Here's how the part is built. I have some questions about the finished solid (model axes, mm). A direction names the side the tool comes from. Round coordinates to 2 decimals unless told otherwise and drop trailing zeros. Write each loop counter-clockwise with the first axis right and the second up, starting at its lowest first coordinate (ties: lowest second). Pieces come first, ordered by that corner, then holes. Notation, with made-up numbers: (39.25, -37) -> (71.25, -37) arc R22 ccw to (71.25, -9) -> close; hole circle Ø2 at (68, 18). An arc over 180 degrees is marked (long way). Answer in a Markdown table with one row per item.
from build123d import *

# Parameters (mm, degrees)
ESBO_O1_W                                            = 18
ESBO_O1_H                                            = 28.5
RESSALTO_EXTRUS_O1_DEPTH                             = 8
ESCAREADO_PARA_PARAFUSO_COM_CABE_A_ESCAR_D           = 2.4
ESCAREADO_PARA_PARAFUSO_COM_CABE_A_ESCAR_CSINK_D     = 4.4
ESCAREADO_PARA_PARAFUSO_COM_CABE_A_ESCAR_CSINK_ANGLE = 90
CORTE_EXTRUS_O1_DEPTH                                = 4
ESCAREADO_PARA_PARAFUSO_COM_CABE_A_E_3_D             = 2.4
ESCAREADO_PARA_PARAFUSO_COM_CABE_A_E_3_CSINK_D       = 4.4
ESCAREADO_PARA_PARAFUSO_COM_CABE_A_E_3_CSINK_ANGLE   = 90
CORTE_EXTRUS_O2_DEPTH                                = 35.644624403
FILETE1_R                                            = 5
CHANFRO1_SIZE                                        = 1
CHANFRO2_SIZE                                        = 1
BROCA_DE_ROSQUEAR_PARA_TARRAXA_DE_M21_D              = 1.6


# Read off the part's stored shape, not the designer's step: Escareado para parafuso com cabeça escareada chata de M21
with BuildPart() as part:
    # Esboço1 → Ressalto-extrusão1 (new body)
    with BuildSketch(Plane(origin=(0, 0, 0), x_dir=(1, 0, 0), z_dir=(0, 1, 0))):
        with Locations((9, 14.25)):
            Rectangle(ESBO_O1_W, ESBO_O1_H)
        with BuildLine():
            Line((5, 11.5), (13, 11.5))
            ThreePointArc((13, 11.5), (14.414213562, 12.085786438), (15, 13.5))
            Line((15, 13.5), (15, 16.5))
            ThreePointArc((15, 16.5), (14.414213562, 17.914213562), (13, 18.5))
            Line((13, 18.5), (5, 18.5))
            ThreePointArc((5, 18.5), (3.585786438, 17.914213562), (3, 16.5))
            Line((3, 16.5), (3, 13.5))
            ThreePointArc((3, 13.5), (3.585786438, 12.085786438), (5, 11.5))
        make_face(mode=Mode.SUBTRACT)
    extrude(amount=RESSALTO_EXTRUS_O1_DEPTH)

    # Escareado para parafuso com cabe_a escar (through all)
    with Locations(Plane(origin=(5, 8, -26), x_dir=(0, 0, 1), z_dir=(0, 1, 0))):
        with Locations((0, 0), (0, 8)):
            CounterSinkHole(ESCAREADO_PARA_PARAFUSO_COM_CABE_A_ESCAR_D / 2, ESCAREADO_PARA_PARAFUSO_COM_CABE_A_ESCAR_CSINK_D / 2, counter_sink_angle=ESCAREADO_PARA_PARAFUSO_COM_CABE_A_ESCAR_CSINK_ANGLE)

    # Esboço10 → Corte-extrusão1 (cut)
    with BuildSketch(Plane.XZ):
        Polygon((0, -28.5), (18, -28.5), (18, -23.5), (15, -23.5), (15, -15), (3, -15), (3, -23.5), (0, -23.5), align=None)
    extrude(amount=-CORTE_EXTRUS_O1_DEPTH, mode=Mode.SUBTRACT)

    # Escareado para parafuso com cabe_a e 2 o → Escareado para parafuso com cabe_a e 2 (revolve, cut)
    with BuildSketch(Plane(origin=(0, 2, -21.5), x_dir=(0, 1, 0), z_dir=(0, 0, -1))):
        Polygon((2.2, 18), (0, 18), (0, 15), (1.2, 15), (1.2, 17), align=None)
    revolve(axis=Axis((0, 2, -21.5), (1, 0, 0)), mode=Mode.SUBTRACT)

    # Escareado para parafuso com cabe_a e 3 (through all)
    with Locations(Plane(origin=(0, 2, -21.5), x_dir=(0, 0, -1), z_dir=(-1, 0, 0))):
        with Locations((0, 0)):
            CounterSinkHole(ESCAREADO_PARA_PARAFUSO_COM_CABE_A_E_3_D / 2, ESCAREADO_PARA_PARAFUSO_COM_CABE_A_E_3_CSINK_D / 2, counter_sink_angle=ESCAREADO_PARA_PARAFUSO_COM_CABE_A_E_3_CSINK_ANGLE)

    # Esboço15 → Corte-extrusão2 (cut, through all)
    with BuildSketch(Plane(origin=(0, 8, 0), x_dir=(1, 0, 0), z_dir=(0, 1, 0))):
        Polygon((0, 0), (4, 0), (0, 11.5), align=None)
        Polygon((18, 0), (18, 11.5), (14, 0), align=None)
    extrude(amount=-CORTE_EXTRUS_O2_DEPTH, mode=Mode.SUBTRACT)

    # Filete1
    filete1_edges = [part.edges().sort_by_distance(p)[0] for p in [
        (0, 4, -11.5),
        (4, 4, 0),
        (14, 4, 0),
        (18, 4, -11.5),
    ]]
    fillet(filete1_edges, radius=FILETE1_R)

    # Chanfro1
    chanfro1_edges = [part.edges().sort_by_distance(p)[0] for p in [
        (16.445137101, 8, -7.029769164),
        (0, 8, -20.422372289),
        (1.554862899, 8, -7.029769164),
        (9, 8, 0),
        (18, 8, -20.422372289),
        (13.342458661, 8, -0.924891681),
        (0.069867146, 8, -11.511803979),
        (4.657541339, 8, -0.924891681),
        (17.930132854, 8, -11.511803979),
        (3.585786438, 8, -12.085786438),
        (14.414213562, 8, -17.914213562),
        (9, 8, -18.5),
        (3.585786438, 8, -17.914213562),
        (3, 8, -15),
        (9, 8, -11.5),
        (14.414213562, 8, -12.085786438),
        (15, 8, -15),
    ]]
    chamfer(chanfro1_edges, length=CHANFRO1_SIZE)

    # Chanfro2
    # the kernel refuses this chamfer: 1 mm, written as the material it takes off along each edge
    with BuildSketch(Plane(origin=(0, 0, -26.071682988), x_dir=(0.9996219169112968, -0.027495876610586372, 0), z_dir=(0, 0, 1)), Plane(origin=(18, 0, -19.844832151), x_dir=(-0.9996219169112968, -0.02749587661058639, 0), z_dir=(0, 0, -1))) as chanfro2_piece_1:
        Polygon((CHANFRO2_SIZE * 0.999621916911, CHANFRO2_SIZE * 0.0274958766106), (-CHANFRO2_SIZE * 0.0274958766106, CHANFRO2_SIZE * 0.999621916911), (0, 0), align=None)
    extrude(amount=6.226850837, mode=Mode.SUBTRACT)
    with BuildSketch(Plane(origin=(17.722483984, 0, -10.702141453), x_dir=(-0.94413969843999, -0.02749587661058639, -0.32839641684869236), z_dir=(-0.3285206249412729, 0, 0.944496796706159)), Plane(origin=(2.832209783, 0, -3.357396875), x_dir=(0.9441396984399901, -0.02749587661058552, -0.32839641684869225), z_dir=(-0.32852062494127277, 0, -0.9444967967061592))) as chanfro2_piece_2:
        Polygon((CHANFRO2_SIZE * 0.999621916911, -CHANFRO2_SIZE * 0.0274958766106), (-CHANFRO2_SIZE * 0.0274958766106, -CHANFRO2_SIZE * 0.999621916911), (0, 0), align=None)
    extrude(amount=7.776357318, mode=Mode.SUBTRACT)
    with BuildSketch(Plane(origin=(18, 0, -12.344744577), x_dir=(-0.9996219169112968, -0.02749587661058639, 0), z_dir=(0, 0, -1)), Plane(origin=(0, 0, -23.155167849), x_dir=(0.9996219169112968, -0.027495876610586372, 0), z_dir=(0, 0, 1))) as chanfro2_piece_3:
        Polygon((CHANFRO2_SIZE * 0.999621916911, CHANFRO2_SIZE * 0.0274958766106), (-CHANFRO2_SIZE * 0.0274958766106, CHANFRO2_SIZE * 0.999621916911), (0, 0), align=None)
    extrude(amount=10.810423272, mode=Mode.SUBTRACT)
    with BuildSketch(Plane(origin=(7.554693766, 0, 0), x_dir=(0, 0.9996219169112968, 0.027495876610586372), z_dir=(1, 0, 0))) as chanfro2_piece_4:
        Polygon((CHANFRO2_SIZE * 0.999621916911, -CHANFRO2_SIZE * 0.0274958766106), (-CHANFRO2_SIZE * 0.0274958766106, -CHANFRO2_SIZE * 0.999621916911), (0, 0), align=None)
    extrude(amount=2.890612468, mode=Mode.SUBTRACT)
    with BuildSketch(Plane(origin=(10.445306234, 0, -5), x_dir=(0, 0, 1), z_dir=(-1, 0, 0))) as chanfro2_piece_5:
        Polygon((5 - CHANFRO2_SIZE, 0), (5, CHANFRO2_SIZE), (5, 0), align=None)
    revolve(axis=Axis((10.445306234, 0, -5), (0, 1, 0)), revolution_arc=70.820991974, mode=Mode.SUBTRACT)
    with BuildSketch(Plane(origin=(5, 0, -12.344744577), x_dir=(-0.944496796706159, 0, 0.32852062494127277), z_dir=(0.32852062494127277, 0, 0.944496796706159))) as chanfro2_piece_6:
        Polygon((5 - CHANFRO2_SIZE, 0), (5, -CHANFRO2_SIZE), (5, 0), align=None)
    revolve(axis=Axis((5, 0, -12.344744577), (0, -1, 0)), revolution_arc=19.179008026, mode=Mode.SUBTRACT)
    with BuildSketch(Plane(origin=(7.554693766, 0, -5), x_dir=(0, 0, 1), z_dir=(1, 0, 0))) as chanfro2_piece_7:
        Polygon((5, -CHANFRO2_SIZE), (5 - CHANFRO2_SIZE, 0), (5, 0), align=None)
    revolve(axis=Axis((7.554693766, 0, -5), (0, -1, 0)), revolution_arc=70.820991974, mode=Mode.SUBTRACT)
    with BuildSketch(Plane(origin=(13, 0, -12.344744577), x_dir=(0.9444967967061589, 0, 0.3285206249412729), z_dir=(-0.3285206249412729, 0, 0.9444967967061589))) as chanfro2_piece_8:
        Polygon((5 - CHANFRO2_SIZE, 0), (5, CHANFRO2_SIZE), (5, 0), align=None)
    revolve(axis=Axis((13, 0, -12.344744577), (0, 1, 0)), revolution_arc=19.179008026, mode=Mode.SUBTRACT)

    # Broca de rosquear para tarraxa de M21 (through all)
    with Locations(Plane(origin=(6, 8, -7), x_dir=(0, 0, 1), z_dir=(0, 1, 0))):
        with Locations((0, 0), (0, 6)):
            Hole(BROCA_DE_ROSQUEAR_PARA_TARRAXA_DE_M21_D / 2)


solid = part.part
1) For pin 1 (2.5 mm diameter, centred on x = 1, y = 2, fed in from -Z); pin 2 (1.4 mm diameter, centred on y = 2, z = -21.5, fed in from -X); pin 3 (9.5 mm diameter, centred on x = 10, z = -23, fed in from -Y); pin 4 (4 mm diameter, centred on y = 2, z = -21.5, fed in from -X), each with a flat end and sliding along its axis, tell me the tip position at first contact or that it passes through.
Response:
| item | result |
|---|---|
| pin 1 | stops at z = -23.5 |
| pin 2 | passes through |
| pin 3 | stops at y = 4 |
| pin 4 | stops at x = 0.2 |
2) I want a section at B-B, the plane z = -21.5. List the corners of the cut face in (x, y) for me.
Response:
| item | result |
|---|---|
| outline | (0, 4.2) -> (1, 3.2) -> (3, 3.2) -> (3, 4) -> (15, 4) -> (15, 3.2) -> (17, 3.2) -> (18, 4.2) -> (18, 7) -> (17, 8) -> (1, 8) -> (0, 7) -> close; (0.6, 0.4) -> (1, 0) -> (3, 0) -> (3, 0.8) -> (1, 0.8) -> close; (15, 0) -> (17, 0) -> (17.4, 0.4) -> (17, 0.8) -> (15, 0.8) -> close |
3) Which directions (+Z, -Z, +X, -X, +Y, -Y) give clear straight access to the entire face, cutting with the end or side of a thin tool? Please do faces 4 (the face through (3.297, 7.382, -11.834)), 5 (the face through (3.6, 5.48, -17.93)), 6 (the face through (3, 3, -17)).
Response:
| item | result |
|---|---|
| face 4 | +Y |
| face 5 | +Y, -Y |
| face 6 | -Y |
4) We'd pull the mould along X, two halves only. Please class faces 1 (the face through (14.666, 7.382, -11.797)), 2 (the face through (16, 7.49, -7.24)), 3 (the face through (9, 0, -10)): +X half, -X half, draft (parallel to the pull), parting line (faces both ways), or undercut.
Response:
| item | result |
|---|---|
| face 1 | undercut |
| face 2 | +X half |
| face 3 | draft |
5) I want a section at A-A, the plane y = 2. List the corners of the cut face in (x, z) for me.
Response:
| item | result |
|---|---|
| outline | (0, -19.3) -> (1, -20.3) -> (3, -20.3) -> (3, -13.5) arc R2 cw to (5, -11.5) -> (13, -11.5) arc R2 cw to (15, -13.5) -> (15, -20.3) -> (17, -20.3) -> (18, -19.3) -> (18, -12.34) arc R5 ccw to (17.72, -10.7) -> (15.17, -3.36) arc R5 ccw to (10.45, 0) -> (7.55, 0) arc R5 ccw to (2.83, -3.36) -> (0.28, -10.7) arc R5 ccw to (0, -12.34) -> close; (0.2, -23.5) -> (3, -23.5) -> (3, -22.7) -> (1, -22.7) -> close; (15, -23.5) -> (17.8, -23.5) -> (17, -22.7) -> (15, -22.7) -> close; hole circle Ø1.6 at (6, -7); hole circle Ø1.6 at (12, -7) |
6) I want a section at C-C, the plane z = -14. List the corners of the cut face in (x, y) for me, and give its area (3 significant figures).
Response:
| item | result |
|---|---|
| outline | (0, 1) -> (1, 0) -> (3, 0) -> (3, 7) -> (2, 8) -> (1, 8) -> (0, 7) -> close; (15, 0) -> (17, 0) -> (18, 1) -> (18, 7) -> (17, 8) -> (16, 8) -> (15, 7) -> close |
| area | 45.0 mm^2 |
7) I want a section at D-D, the plane x = 13.5. Count the separate pieces of the cut face and the enclosed holes in it, and give its area (3 significant figures).
Response:
| item | result |
|---|---|
| separate pieces | 3 |
| enclosed holes | 0 |
| area | 112 mm^2 |
8) I need wall thicknesses on line 1 (X direction, y = 6, z = -26); line 2 (Z direction, x = 13, y = 4.95); line 3 (Y direction, x = 1.65, z = -21.5). Which ranges of each line are inside material? Lowest first, please. Write a range as [from, to].
Response:
| item | result |
|---|---|
| line 1 | x = [0, 3.8], [6.2, 11.8], [14.2, 18] |
| line 2 | z = [-28.5, -27.2], [-24.8, -18.5], [-11.5, -0.7] |
| line 3 | y = [0, 0.8], [3.2, 8] |
